```python
from build123d import *

# Parameters (mm, degrees)
F2_DEPTH = 11.938
F3_DEPTH = 25.4
F5_DEPTH = 72.644
F6_R     = 7.860553
F7_DEPTH = 35.306


with BuildPart() as f2:
    # F1 (on Top) → F2 (new body)
    with BuildSketch(Plane.XY):
        Polygon((50.910734, 0), (-55.442028, 0), (-55.442028, -53.830672), (50.910734, -53.498318), align=None)
    extrude(amount=F2_DEPTH)

    # F0 (on Front) → F3 (join)
    with BuildSketch(Plane.XZ):
        Polygon((-54.879387, 19.324376), (-54.879387, 0), (50.584481, 0), (49.630058, 19.324376), (19.565694, 35.072376), (-24.815029, 35.072376), align=None)
    extrude(amount=F3_DEPTH)

    # F4 (on Front) → F5 (cut)
    with BuildSketch(Plane.XZ):
        Polygon((33.436544, 5.434085), (-38.706463, 5.434085), (-33.109158, 0), (27.839245, 0), align=None)
    extrude(amount=F5_DEPTH, mode=Mode.SUBTRACT)

    # F6 (on Top) → F7 (cut)
    with BuildSketch(Plane.XY):
        with Locations((0, -39.10695)):
            Circle(F6_R)
    extrude(amount=F7_DEPTH, mode=Mode.SUBTRACT)


solid = f2.part
```
CAD build for the part. Positions are in the model's coordinates, mm. A direction names the side the tool comes from. Round coordinates to 2 decimals unless told otherwise and drop trailing zeros. Loops run counter-clockwise (first coordinate to the right, second up) from the corner with the lowest first, then second, coordinate; pieces in that order, holes last. Notation, with made-up numbers: M 29,46 L 66,46 A14 ccw 66,50 Z; hole C 65,34 d10. An arc over 180 degrees is marked long. Use a Markdown table: item, result. Add a question column.
(1) Flat gauge pins, fed straight in: pin 1 (5 mm diameter, centred on x = -26.5, z = 22.5, fed in from -Y); pin 2 (8 mm diameter, centred on x = 31, y = -21, fed in from -Z); pin 3 (20.5 mm diameter, centred on x = 0, y = -39.11, fed in from -Z); pin 4 (5 mm diameter, centred on y = -13.5, z = 17.5, fed in from +X). Where does each tip first touch, or does it go through?
(2) Cut at B-B (y = -18.5). Give the cut face in (x, z).
(3) Drill centre lines: line 1 (Z direction, x = -23, y = -11.5); line 2 (Z direction, x = -5.5, y = -33); line 3 (X direction, y = -7.5, z = 19). Where is each one in solid material? Low to high.
(4) Pull direction Z, two halves, no side cores. Call faces 5 (the face through (34.808, -12.522, 27.088)), 6 (the face through (-35.95, -26.51, 2.76)), 7 (the face through (50.911, -27, 6)): +Z half, -Z half, draft (parallel to the pull), parting line (faces both ways), or undercut.
(5) Cut at C-C (x = 0). Give the cut face in (y, z), and give its area (3 significant figures).
(6) Cut at D-D (y = -45). Give the cut face in (x, z).
(7) Cut at A-A (z = 4). Give the cut face in (x, y), and give its area (3 significant figures).
(8) Which spindle directions (+Z, -Z, +X, -X, +Y, -Y) get a long thin tool onto all of the face, cutting with end or side? Do faces 1 (the face through (-54.879, -13, 16)), 2 (the face through (-3, -25.4, 21)), 3 (the face through (-2, -27, 5.434)), 4 (the face through (-55.442, -27, 6)). Say none if no direction does.
Geometry says:
| question | item | result |
|---|---|---|
| 1 | pin 1 | stops at y = -25.4 |
| 1 | pin 2 | stops at z = 0 |
| 1 | pin 3 | stops at z = 5.43 |
| 1 | pin 4 | stops at x = 49.84 |
| 2 | outline | M -55.44,0 L -33.11,0 L -38.71,5.43 L 33.44,5.43 L 27.84,0 L 50.91,0 L 50.91,11.94 L 49.99,11.94 L 49.63,19.32 L 19.57,35.07 L -24.82,35.07 L -54.88,19.32 L -54.88,11.94 L -55.44,11.94 Z |
| 3 | line 1 | z = 5.43 to 35.07 |
| 3 | line 2 | z = 5.43 to 11.94 |
| 3 | line 3 | x = -54.88 to 49.65 |
| 4 | face 5 | +Z half |
| 4 | face 6 | undercut |
| 4 | face 7 | draft |
| 5 | outline | M -53.66,5.43 L -46.97,5.43 L -46.97,11.94 L -53.66,11.94 Z; M -31.25,5.43 L 0,5.43 L 0,35.07 L -25.4,35.07 L -25.4,11.94 L -31.25,11.94 Z |
| 5 | area | 834 mm² |
| 6 | outline | M -55.44,0 L -33.11,0 L -38.71,5.43 L -5.2,5.43 L -5.2,11.94 L -55.44,11.94 Z; M 5.2,5.43 L 33.44,5.43 L 27.84,0 L 50.91,0 L 50.91,11.94 L 5.2,11.94 Z |
| 7 | outline | M -55.44,-53.83 L -37.23,-53.77 L -37.23,0 L -55.44,0 Z; M 31.96,-53.56 L 50.91,-53.5 L 50.91,0 L 31.96,0 Z |
| 7 | area | 1,990 mm² |
| 8 | face 1 | +Z, -X, +Y, -Y |
| 8 | face 2 | +Z, +X, -X, -Y |
| 8 | face 3 | +Y, -Y |
| 8 | face 4 | +Z, -Z, -X, +Y, -Y |
